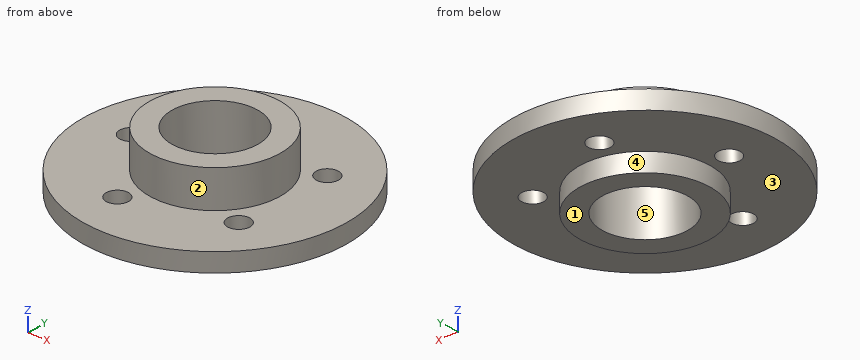
Autodesk Inventor part; units mm, degrees
ref_plane "YZ Plane" through (0, 0, 0) normal (1, 0, 0) x (0, 1, 0)
ref_plane "XZ Plane" through (0, 0, 0) normal (0, 1, 0) x (-1, 0, 0)
ref_plane "XY Plane" through (0, 0, 0) normal (0, 0, 1) x (1, 0, 0)
sketch "Sketch1" plane through (0, 0, 0) normal (0, 0, 1) x (1, 0, 0)
  line L0 (-25.1788, 61.8531) -> (-25.1788, 68.2031)
  line L1 (-13.5921, 60.3277) -> (-11.9486, 66.4613)
  line L2 (-2.7951, 55.8554) -> (0.3799, 61.3547)
  line L3 (6.4766, 48.741) -> (10.9667, 53.2312)
  line L4 (13.591, 39.4694) -> (19.0902, 42.6444)
  line L5 (18.0633, 28.6723) -> (24.1969, 30.3158)
  line L6 (19.5887, 17.0856) -> (25.9387, 17.0856)
  line L7 (18.0633, 5.4989) -> (24.1969, 3.8554)
  line L8 (13.591, -5.2981) -> (19.0902, -8.4731)
  line L9 (6.4766, -14.5698) -> (10.9667, -19.0599)
  line L10 (-2.7951, -21.6842) -> (0.3799, -27.1834)
  line L11 (-13.5921, -26.1565) -> (-11.9486, -32.2901)
  line L12 (-25.1788, -27.6819) -> (-25.1788, -34.0319)
  line L13 (-36.7655, -26.1565) -> (-38.409, -32.2901)
  line L14 (-47.5626, -21.6842) -> (-50.7376, -27.1834)
  line L15 (-56.8342, -14.5698) -> (-61.3243, -19.0599)
  line L16 (-63.9486, -5.2981) -> (-69.4479, -8.4731)
  line L17 (-68.4209, 5.4989) -> (-74.5545, 3.8554)
  line L18 (-69.9463, 17.0856) -> (-76.2963, 17.0856)
  line L19 (-68.4209, 28.6723) -> (-74.5545, 30.3158)
  line L20 (-63.9486, 39.4694) -> (-69.4479, 42.6444)
  line L21 (-56.8342, 48.741) -> (-61.3243, 53.2312)
  line L22 (-47.5626, 55.8554) -> (-50.7376, 61.3547)
  line L23 (-36.7655, 60.3277) -> (-38.409, 66.4613)
  arc A0 (-38.409, 66.4613) -> (-25.1788, 68.2031) centre (-31.8994, 68.1336) ccw
  arc A1 (-25.1788, 68.2031) -> (-11.9486, 66.4613) centre (-18.4582, 68.1336) ccw
  arc A2 (-11.9486, 66.4613) -> (0.3799, 61.3547) centre (-5.475, 64.6547) ccw
  arc A3 (0.3799, 61.3547) -> (10.9667, 53.2312) centre (6.1654, 57.9342) ccw
  arc A4 (10.9667, 53.2312) -> (19.0902, 42.6444) centre (15.6697, 48.4298) ccw
  arc A5 (19.0902, 42.6444) -> (24.1969, 30.3158) centre (22.3903, 36.7894) ccw
  arc A6 (24.1969, 30.3158) -> (25.9387, 17.0856) centre (25.8692, 23.8062) ccw
  arc A7 (25.9387, 17.0856) -> (24.1969, 3.8554) centre (25.8692, 10.365) ccw
  arc A8 (24.1969, 3.8554) -> (19.0902, -8.4731) centre (22.3903, -2.6182) ccw
  arc A9 (19.0902, -8.4731) -> (10.9667, -19.0599) centre (15.6697, -14.2586) ccw
  arc A10 (10.9667, -19.0599) -> (0.3799, -27.1834) centre (6.1654, -23.7629) ccw
  arc A11 (0.3799, -27.1834) -> (-11.9486, -32.2901) centre (-5.475, -30.4835) ccw
  arc A12 (-11.9486, -32.2901) -> (-25.1788, -34.0319) centre (-18.4582, -33.9623) ccw
  arc A13 (-25.1788, -34.0319) -> (-38.409, -32.2901) centre (-31.8994, -33.9623) ccw
  arc A14 (-38.409, -32.2901) -> (-50.7376, -27.1834) centre (-44.8826, -30.4835) ccw
  arc A15 (-50.7376, -27.1834) -> (-61.3243, -19.0599) centre (-56.523, -23.7629) ccw
  arc A16 (-61.3243, -19.0599) -> (-69.4479, -8.4731) centre (-66.0273, -14.2586) ccw
  arc A17 (-69.4479, -8.4731) -> (-74.5545, 3.8554) centre (-72.7479, -2.6182) ccw
  arc A18 (-74.5545, 3.8554) -> (-76.2963, 17.0856) centre (-76.2268, 10.365) ccw
  arc A19 (-76.2963, 17.0856) -> (-74.5545, 30.3158) centre (-76.2268, 23.8062) ccw
  arc A20 (-74.5545, 30.3158) -> (-69.4479, 42.6444) centre (-72.7479, 36.7894) ccw
  arc A21 (-69.4479, 42.6444) -> (-61.3243, 53.2312) centre (-66.0273, 48.4298) ccw
  arc A22 (-61.3243, 53.2312) -> (-50.7376, 61.3547) centre (-56.523, 57.9342) ccw
  arc A23 (-50.7376, 61.3547) -> (-38.409, 66.4613) centre (-44.8826, 64.6547) ccw
  circle A24 centre (-25.1788, 17.0856) radius 44.7675
  point P0 (0, 0)
  dimension "d36" = 89.535
  dimension "d8" = 360
extrude "Extrusion1" add sketch "Sketch1" along normal blind 6.35 contours A24
sketch "Sketch2" plane through (-25.1788, 17.0856, 0) normal (0, 0, -1) x (-1, 0, 0)
  circle A0 centre (-23.7729, 17.272) radius 3.81
  circle A1 centre (0, 0) radius 44.7675
  circle A2 centre (9.0804, 27.9467) radius 3.81
  circle A3 centre (29.3849, 0) radius 3.81
  circle A4 centre (9.0804, -27.9467) radius 3.81
  circle A5 centre (-23.7729, -17.272) radius 3.81
  point P0 (-25.1788, -17.0856)
  dimension "d15" = 360
  dimension "d17" = 17.272
  dimension "d19" = 0
  dimension "d20" = 7.62
hole "Hole1" at (-1.4059, 34.3576, 0) at (-1.4059, -0.1864, 0) at (-34.2592, 45.0323, 0) at (-34.2592, -10.8611, 0) at (-54.5637, 17.0856, 0) direction (0, 0, 1) diameter 7.62 end through all
sketch "Sketch3" plane through (-25.1788, 17.0856, 0) normal (0, 0, -1) x (-1, 0, 0)
  point P0 (-25.1788, -17.0856)
sketch "Sketch4" plane through (-25.1788, 17.0856, 0) normal (0, 0, -1) x (-1, 0, 0)
  point P0 (-25.1788, -17.0856)
sketch "Sketch6" plane through (-25.1788, 17.0856, 6.35) normal (0, 0, 1) x (1, 0, 0)
  circle A0 centre (0, 0) radius 14.605
  point P0 (25.1788, -17.0856)
  dimension "d48" = 29.21
sketch "Sketch7" plane through (-25.1788, 17.0856, 6.35) normal (0, 0, 1) x (1, 0, 0)
  circle A0 centre (0, 0) radius 22.225
  point P0 (25.1788, -17.0856)
  dimension "d51" = 44.45
extrude "Extrusion4" add sketch "Sketch7" along normal mid plane 25.4
extrude "Extrusion5" cut sketch "Sketch6" along normal through all both and the other way through all
properties part number "PVC motor gear"
Build history of the part. All positions in model axes, mm. Face numbers are marked on the shaded views. A direction names the side the tool comes from. Round coordinates to 2 decimals unless told otherwise and drop trailing zeros. Write each loop counter-clockwise with the first axis right and the second up, starting at its lowest first coordinate (ties: lowest second). Pieces come first, ordered by that corner, then holes.
1) 3-axis set-ups, long thin cutter, end or side, ignore diameter. For the marked faces 1 and 2: which of +Z, -Z, +X, -X, +Y, -Y reach the whole face in a straight line?
2) Mould opens along Y. For the marked faces 3, 4 and 5 say: +Y half, -Y half, draft (parallel to the pull), parting line (faces both ways), or undercut.
3) Band-saw the part on C-C, the plane z = 13.5. List the corners of the cut face in (x, y) (3 decimals), and give its area (3 significant figures).
4) Band-saw the part on D-D, the plane y = -11.5. List the corners of the cut face in (x, z), and give its area (3 significant figures).
5) Band-saw the part on B-B, the plane y = 34. List the corners of the cut face in (x, z), and give its area (3 significant figures).
6) Pin check, flat tips, straight feed: pin 1 (1.5 mm diameter, centred on x = 0.5, y = 4.5, fed in from +Z); pin 2 (3 mm diameter, centred on x = -43, z = 9, fed in from -Y); pin 3 (6 mm diameter, centred on x = -1.41, y = 34.36, fed in from +Z); pin 4 (8 mm diameter, centred on x = -56, y = 4.5, fed in from -Z). Stop position of each tip, or through.
7) Drill centre lines: probe 1 along X at (y, z) = (19, 6.25); probe 2 along Z at (x, y) = (-0.5, 28); probe 3 along Y at (x, z) = (-25, 5.5). Where is each one in solid material? Low to high.
8) Band-saw the part on A-A, the plane x = -27. List the corners of the cut face in (y, z).
Ans:
1. face 1: -Z, +X, -X, +Y, -Y
1. face 2: +Z
2. face 3: draft
2. face 4: parting line
2. face 5: undercut
3. outline: circle Ø44.45 at (-25.179, 17.086); hole circle Ø29.21 at (-25.179, 17.086)
3. area: 882 mm2
4. outline: (-59.63, 0) - (-38.02, 0) - (-38.02, 6.35) - (-59.63, 6.35) - close; (-30.5, 0) - (9.27, 0) - (9.27, 6.35) - (-30.5, 6.35) - close
4. area: 390 mm2
5. outline: (-66.63, 0) - (-39.6, 0) - (-39.6, -6.35) - (-10.76, -6.35) - (-10.76, 0) - (-5.2, 0) - (-5.2, 6.35) - (-10.76, 6.35) - (-10.76, 19.05) - (-39.6, 19.05) - (-39.6, 6.35) - (-66.63, 6.35) - close; (2.39, 0) - (16.27, 0) - (16.27, 6.35) - (2.39, 6.35) - close
5. area: 1,030 mm2
6. pin 1: stops at z = 6.35
6. pin 2: stops at y = 2
6. pin 3: passes through
6. pin 4: stops at z = 0
7. probe 1: x = -69.91 to -57.86, -51.27 to -39.66, -10.7 to 19.55
7. probe 2: z = 0 to 6.35
7. probe 3: y = -27.68 to 2.48, 31.69 to 61.85
8. outline: (-27.64, 0) - (-5.06, 0) - (-5.06, -6.35) - (2.59, -6.35) - (2.59, 19.05) - (-5.06, 19.05) - (-5.06, 6.35) - (-27.64, 6.35) - close; (31.58, -6.35) - (39.24, -6.35) - (39.24, 0) - (61.82, 0) - (61.82, 6.35) - (39.24, 6.35) - (39.24, 19.05) - (31.58, 19.05) - close
